CAD build for the part. Positions are in the model's coordinates, mm. Face numbers are marked on the shaded views. A direction names the side the tool comes from. Round coordinates to 2 decimals unless told otherwise and drop trailing zeros. Loops run counter-clockwise (first coordinate to the right, second up) from the corner with the lowest first, then second, coordinate; pieces in that order, holes last. Notation, with made-up numbers: M 31,33.25 L 77,33.25 A14 ccw 77,46.25 Z; hole C -11,49 d1. An arc over 180 degrees is marked long. Use a Markdown table: item, result. Add a question column.
(1) Band-saw the part on C-C, the plane y = 0.45. Write the cut outline in (x, z), and give its area (3 significant figures).
(2) Flat gauge pin, fed straight in: P1, Ø0.8, axis at x = 5.5, y = 1.5, coming from the -Z side. Where does the tip first touch, or does it go through?
(3) Two-plate mould, pull along X, no slides. Class the marked faces 3, 4 and 5: released by +X, released by -X, zero draft, split by the parting line, or undercut.
(4) Which spindle directions (+Z, -Z, +X, -X, +Y, -Y) get a long thin tool onto all of the face, cutting with end or side? Do the marked faces 1 and 2. Say none if no direction does.
(5) Wall check: L1, parallel to Z at x = 7.5, y = 1.9; L2, parallel to X at y = 1.2, z = 3.5; L3, parallel to Z at x = 1, y = 1.5. Give the ranges that are in metal, low to high.
(6) Band-saw the part on D-D, the plane z = -0.5. Write the cut outline in (x, y) (3 decimals).
(7) Band-saw the part on A-A, the plane x = 6.35. Write the cut outline in (y, z).
(8) Band-saw the part on B-B, the plane z = 4.25. Write the cut outline in (x, y) (3 decimals).
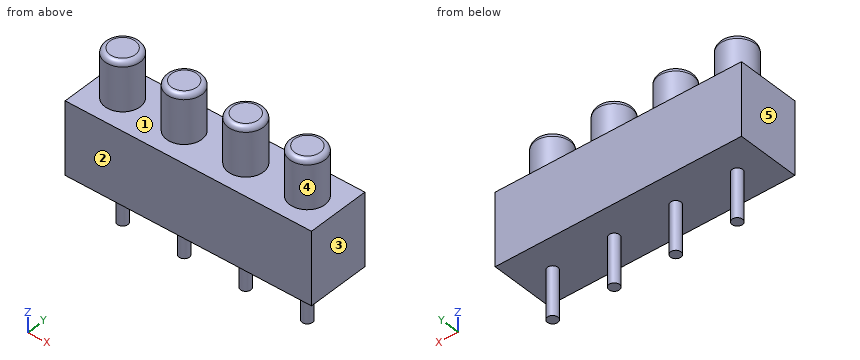
from build123d import *

# Parameters (mm, degrees)
SKETCH_1_W      = 10.16
SKETCH_1_H      = 2.59
EXTRUDE_1_DEPTH = 3
SKETCH_2_R      = 0.725
EXTRUDE_2_DEPTH = 2
SKETCH_3_R      = 0.215
EXTRUDE_3_DEPTH = 2
FILLET_1_R      = 0.2


with BuildPart() as part:
    # Эскиз1 → Бобышка-Вытянуть1 (new body)
    with BuildSketch(Plane.XY):
        with Locations((5.08, 1.295)):
            Rectangle(SKETCH_1_W, SKETCH_1_H)
    extrude(amount=EXTRUDE_1_DEPTH)

    # Эскиз2 → Бобышка-Вытянуть2 (add)
    with BuildSketch(Plane.XY.offset(3)):
        with Locations(Location((1.27, 1.295, 0), (0, 0, 180))):
            Circle(SKETCH_2_R)
        with Locations(Location((3.81, 1.295, 0), (0, 0, 180))):
            Circle(SKETCH_2_R)
        with Locations(Location((6.35, 1.295, 0), (0, 0, 180))):
            Circle(SKETCH_2_R)
        with Locations(Location((8.89, 1.295, 0), (0, 0, 180))):
            Circle(SKETCH_2_R)
    extrude(amount=EXTRUDE_2_DEPTH)

    # Эскиз3 → Бобышка-Вытянуть3 (add)
    with BuildSketch(Plane(origin=(0, 0, 0), x_dir=(-1, 0, 0), z_dir=(0, 0, -1))):
        with Locations((-1.27, 1.295)):
            Circle(SKETCH_3_R)
        with Locations((-3.81, 1.295)):
            Circle(SKETCH_3_R)
        with Locations((-6.35, 1.295)):
            Circle(SKETCH_3_R)
        with Locations((-8.89, 1.295)):
            Circle(SKETCH_3_R)
    extrude(amount=EXTRUDE_3_DEPTH)

    # Скругление1
    fillet_1_edges = [part.edges().sort_by_distance(p)[0] for p in [
        (1.995, 1.295, 5),
        (4.535, 1.295, 5),
        (7.075, 1.295, 5),
        (9.615, 1.295, 5),
    ]]
    fillet(fillet_1_edges, radius=FILLET_1_R)


solid = part.part
Return value:
| question | item | result |
|---|---|---|
| 1 | outline | M 0,0 L 10.16,0 L 10.16,3 L 0,3 Z |
| 1 | area | 30.5 mm^2 |
| 2 | P1 | z = 0 |
| 3 | face 3 | released by +X |
| 3 | face 4 | undercut |
| 3 | face 5 | released by -X |
| 4 | face 1 | +Z |
| 4 | face 2 | +Z, -Z, +X, -X, -Y |
| 5 | L1 | 0 to 3 |
| 5 | L2 | 0.55 to 1.99, 3.09 to 4.53, 5.63 to 7.07, 8.17 to 9.61 |
| 5 | L3 | 0 to 5 |
| 6 | outline | C 1.27,1.295 d0.43; C 3.81,1.295 d0.43; C 6.35,1.295 d0.43; C 8.89,1.295 d0.43 |
| 7 | outline | M 0,0 L 1.08,0 L 1.08,-2 L 1.51,-2 L 1.51,0 L 2.59,0 L 2.59,3 L 2.02,3 L 2.02,4.8 A0.2 ccw 1.82,5 L 0.77,5 A0.2 ccw 0.57,4.8 L 0.57,3 L 0,3 Z |
| 8 | outline | C 1.27,1.295 d1.45; C 3.81,1.295 d1.45; C 6.35,1.295 d1.45; C 8.89,1.295 d1.45 |
